```python
from build123d import *

# Parameters (mm, degrees)
BOSS_EXTRUDE1_DEPTH = 125
BOSS_EXTRUDE2_DEPTH = 10
SKETCH3_W           = 900
SKETCH3_H           = 350
SKETCH3_R           = 15
BOSS_EXTRUDE3_DEPTH = 20
SKETCH5_W           = 100
SKETCH5_H           = 540
BOSS_EXTRUDE4_DEPTH = 20
CUT_EXTRUDE1_START  = -676
CUT_EXTRUDE1_DEPTH  = 676


with BuildPart() as part:
    # Sketch1 → Boss-Extrude1 (new, symmetric)
    with BuildSketch(Plane.XY):
        with BuildLine():
            Line((-317, 0), (-305, 0))
            ThreePointArc((-305, 0), (0, -305), (305, 0))
            Line((305, 0), (317, 0))
            ThreePointArc((317, 0), (0, -317), (-317, 0))
        make_face()
    extrude(amount=BOSS_EXTRUDE1_DEPTH, both=True)

    # Sketch2 → Boss-Extrude2 (add, symmetric)
    with BuildSketch(Plane.XY):
        with BuildLine():
            Line((-216.821053663, -231.252309585), (-350, -713.189409477))
            Line((-350, -713.189409477), (350, -713.189409477))
            Line((350, -713.189409477), (216.821053663, -231.252309585))
            ThreePointArc((216.821053663, -231.252309585), (0, -317), (-216.821053663, -231.252309585))
        make_face()
    extrude(amount=BOSS_EXTRUDE2_DEPTH, both=True)

    # Sketch3 → Boss-Extrude3 (add)
    with BuildSketch(Plane.XZ.offset(713.189409477)):
        Rectangle(SKETCH3_W, SKETCH3_H)
        with Locations(Location((-350, 125, 0), (0, 0, 270))):
            Circle(SKETCH3_R, mode=Mode.SUBTRACT)
        with Locations(Location((350, 125, 0), (0, 0, 270))):
            Circle(SKETCH3_R, mode=Mode.SUBTRACT)
        with Locations(Location((-350, -125, 0), (0, 0, 270))):
            Circle(SKETCH3_R, mode=Mode.SUBTRACT)
        with Locations(Location((350, -125, 0), (0, 0, 270))):
            Circle(SKETCH3_R, mode=Mode.SUBTRACT)
    extrude(amount=BOSS_EXTRUDE3_DEPTH)

    # Sketch5 → Boss-Extrude4 (add)
    with BuildSketch(Plane(origin=(-142.067675448, 39.259113542, 0), x_dir=(0, 0, 1), z_dir=(-0.9638741997846356, 0.266357892673614, 0))):
        with Locations((0, -530.650133791)):
            Rectangle(SKETCH5_W, SKETCH5_H)
    boss_extrude4 = extrude(amount=BOSS_EXTRUDE4_DEPTH)

    # Mirror1: Boss-Extrude4 across plane
    add(boss_extrude4.mirror(Plane(origin=(0, 0, 0), x_dir=(0, 0, 1), z_dir=(1, 0, 0))))

    # Sketch6 → Cut-Extrude1 (cut)
    with BuildSketch(Plane(origin=(0, 0, -125), x_dir=(-1, 0, 0), z_dir=(0, 0, -1)).offset(CUT_EXTRUDE1_START)):
        with BuildLine():
            Line((-305, 0), (305, 0))
            ThreePointArc((305, 0), (0, -305), (-305, 0))
        make_face()
    extrude(amount=CUT_EXTRUDE1_DEPTH, mode=Mode.SUBTRACT)


solid = part.part
```
CAD build for the part. Positions are in the model's coordinates, mm. A direction names the side the tool comes from. Give positions to 0.01 mm unless a question says otherwise; leave off trailing zeros. Write each loop counter-clockwise with the first axis right and the second up, starting at its lowest first coordinate (ties: lowest second). Pieces come first, ordered by that corner, then holes. Notation, with made-up numbers: M 62.25,30 L 66.25,30 A23 ccw 66.25,68 Z; hole C 81.25,-17.75 d7. An arc over 180 degrees is marked long. Return JSON: item names as keys, results as strings. Group by question number.
(1) Band-saw the part on A-A (z = 77.5). Give the cut face in (x, y), and give its area (3 significant figures).
(2) 3-axis set-ups, long thin cutter, end or side, ignore diameter. For faces 4 (the face through (-5, -522, -10)), 5 (the face through (293, -470, 50)), 6 (the face through (-5, -522, 10)): which of +Z, -Z, +X, -X, +Y, -Y reach the whole face in a straight line?
(3) Band-saw the part on D-D (y = -390). Give the cut face in (x, z).
(4) Drill centre lines: L1, parallel to X at y = -726.25, z = -125; L2, parallel to Y at x = -19, z = -144; L3, parallel to Z at x = 152, y = -556. Where is each one in solid material? Low to high. Write a range as [from, to].
(5) Band-saw the part on C-C (x = 197.5). Give the cut face in (y, z), and give its area (3 significant figures).
(6) Flat gauge pins, fed straight in: pin 1 Ø2 at (x, y) = (224.5, -443.5) entering from +Z; pin 2 Ø8 at (x, y) = (264, -538.5) entering from -Z; pin 3 Ø1.5 at (x, z) = (135.5, -112.5) entering from +Y. Where does each tip first touch, or does it go through?
(7) Mould opens along Y. For faces 1 (the face through (1, -310, -125)), 2 (the face through (-6, -733.189, 2)), 3 (the face through (-282.48, -468.85, -30.28)) say: pulls with the +Y half, pulls with the -Y half, needs draft (parallel to the pull), parting line crosses it, or undercut.
(8) Band-saw the part on B-B (y = -74). Give the cut face in (x, z), and give its area (3 significant figures).
Entries:
{
 "1": {"outline": "M -450,-733.19 L 450,-733.19 L 450,-713.19 L -450,-713.19 Z; M -317,0 A317 ccw 317,0 L 305,0 A305 cw -305,0 Z", "area": "29,700 mm^2"},
 "2": {"face 4": "-Z", "face 5": "+Z, +X", "face 6": "+Z"},
 "3": {"outline": "M -281.44,-50 L -260.69,-50 L -260.69,-10 L 260.69,-10 L 260.69,-50 L 281.44,-50 L 281.44,50 L 260.69,50 L 260.69,10 L -260.69,10 L -260.69,50 L -281.44,50 Z"},
 "4": {"L1": "x = [-450, -365], [-335, 335], [365, 450]", "L2": "y = [-733.19, -713.19]", "L3": "z = [-10, 10]"},
 "5": {"outline": "M -733.19,-175 L -713.19,-175 L -713.19,-10 L -247.96,-10 L -247.96,-125 L -232.42,-125 L -232.42,125 L -247.96,125 L -247.96,10 L -713.19,10 L -713.19,175 L -733.19,175 Z", "area": "20,200 mm^2"},
 "6": {"pin 1": "stops at z = 10", "pin 2": "stops at z = -10", "pin 3": "stops at y = -272.88"},
 "7": {"face 1": "needs draft", "face 2": "pulls with the -Y half", "face 3": "undercut"},
 "8": {"outline": "M -308.24,-125 L -295.89,-125 L -295.89,125 L -308.24,125 Z; M 295.89,-125 L 308.24,-125 L 308.24,125 L 295.89,125 Z", "area": "6,180 mm^2"}
}
